Source: CAD feature listing. Evaluate the final solid. Frame: model axes, mm. A direction names the side the tool comes from. Round coordinates to 2 decimals unless told otherwise and drop trailing zeros. One line per item, written item: value.
Autodesk Inventor part; units mm, degrees
ref_plane "YZ Plane" through (0, 0, 0) normal (1, 0, 0) x (0, 1, 0)
ref_plane "XZ Plane" through (0, 0, 0) normal (0, 1, 0) x (-1, 0, 0)
ref_plane "XY Plane" through (0, 0, 0) normal (0, 0, 1) x (1, 0, 0)
sketch "_____4" plane through (0, 0, 0) normal (0, 0, 1) x (1, 0, 0)
  line L0 (-10, -3) -> (-10, -9)
  arc A0 (-10, -9) -> (-9, -10) centre (-9, -9) ccw
  line L1 (-9, -10) -> (-3, -10)
  line L2 (-3, -10) -> (-3, -8)
  line L3 (-3, -8) -> (-6, -8)
  line L4 (-6, -8) -> (-6, -7.0607)
  line L5 (-6, -7.0607) -> (-2.9393, -4)
  line L6 (-2.9393, -4) -> (-0.6536, -4)
  arc A1 (-0.6536, -4) -> (-0.4036, -3.933) centre (-0.6536, -3.5) ccw
  line L7 (-0.4036, -3.933) -> (0, -3.7)
  line L8 (0, -3.7) -> (0.4036, -3.933)
  arc A2 (0.4036, -3.933) -> (0.9036, -3.933) centre (0.6536, -3.5) ccw
  line L9 (0.9036, -3.933) -> (1.2189, -3.751)
  line L10 (1.2189, -3.751) -> (2.5, -4)
  line L11 (2.5, -4) -> (2.9393, -4)
  line L12 (2.9393, -4) -> (6, -7.0607)
  line L13 (6, -7.0607) -> (6, -8)
  line L14 (6, -8) -> (3, -8)
  line L15 (3, -8) -> (3, -10)
  line L16 (3, -10) -> (9, -10)
  arc A3 (9, -10) -> (10, -9) centre (9, -9) ccw
  line L17 (10, -9) -> (10, -3)
  line L18 (10, -3) -> (8, -3)
  line L19 (8, -3) -> (8, -6)
  line L20 (8, -6) -> (7.0607, -6)
  line L21 (7.0607, -6) -> (4, -2.9393)
  line L22 (4, -2.9393) -> (4, -0.6536)
  arc A4 (4, -0.6536) -> (3.933, -0.4036) centre (3.5, -0.6536) ccw
  line L23 (3.933, -0.4036) -> (3.7, 0)
  line L24 (3.7, 0) -> (3.933, 0.4036)
  arc A5 (3.933, 0.4036) -> (3.933, 0.9036) centre (3.5, 0.6536) ccw
  line L25 (3.933, 0.9036) -> (3.751, 1.2189)
  line L26 (3.751, 1.2189) -> (4, 2.5)
  line L27 (4, 2.5) -> (4, 2.9393)
  line L28 (4, 2.9393) -> (7.0607, 6)
  line L29 (7.0607, 6) -> (8, 6)
  line L30 (8, 6) -> (8, 3)
  line L31 (8, 3) -> (10, 3)
  line L32 (10, 3) -> (10, 9)
  arc A6 (10, 9) -> (9, 10) centre (9, 9) ccw
  line L33 (9, 10) -> (3, 10)
  line L34 (3, 10) -> (3, 8)
  line L35 (3, 8) -> (6, 8)
  line L36 (6, 8) -> (6, 7.0607)
  line L37 (6, 7.0607) -> (2.9393, 4)
  line L38 (2.9393, 4) -> (0.6536, 4)
  arc A7 (0.6536, 4) -> (0.4036, 3.933) centre (0.6536, 3.5) ccw
  line L39 (0.4036, 3.933) -> (0, 3.7)
  line L40 (0, 3.7) -> (-0.4036, 3.933)
  arc A8 (-0.4036, 3.933) -> (-0.9036, 3.933) centre (-0.6536, 3.5) ccw
  line L41 (-0.9036, 3.933) -> (-1.2189, 3.751)
  line L42 (-1.2189, 3.751) -> (-2.5, 4)
  line L43 (-2.5, 4) -> (-2.9393, 4)
  line L44 (-2.9393, 4) -> (-6, 7.0607)
  line L45 (-6, 7.0607) -> (-6, 8)
  line L46 (-6, 8) -> (-3, 8)
  line L47 (-3, 8) -> (-3, 10)
  line L48 (-3, 10) -> (-9, 10)
  arc A9 (-9, 10) -> (-10, 9) centre (-9, 9) ccw
  line L49 (-10, 9) -> (-10, 3)
  line L50 (-10, 3) -> (-8, 3)
  line L51 (-8, 3) -> (-8, 6)
  line L52 (-8, 6) -> (-7.0607, 6)
  line L53 (-7.0607, 6) -> (-4, 2.9393)
  line L54 (-4, 2.9393) -> (-4, 0.6536)
  arc A10 (-4, 0.6536) -> (-3.933, 0.4036) centre (-3.5, 0.6536) ccw
  line L55 (-3.933, 0.4036) -> (-3.7, 0)
  line L56 (-3.7, 0) -> (-3.933, -0.4036)
  arc A11 (-3.933, -0.4036) -> (-3.933, -0.9036) centre (-3.5, -0.6536) ccw
  line L57 (-3.933, -0.9036) -> (-3.751, -1.2189)
  line L58 (-3.751, -1.2189) -> (-4, -2.5)
  line L59 (-4, -2.5) -> (-4, -2.9393)
  line L60 (-4, -2.9393) -> (-7.0607, -6)
  line L61 (-7.0607, -6) -> (-8, -6)
  line L62 (-8, -6) -> (-8, -3)
  line L63 (-8, -3) -> (-10, -3)
extrude "Extrusion1" add sketch "_____4" against normal blind 140
sketch "Sketch2" plane through (0, 0, -140) normal (0, 0, -1) x (-1, 0, 0)
  point P0 (0, 0)
hole "Hole1" at (0, 0, -140) direction (0, 0, 1) diameter 4.2 depth 4000
properties part number "KNFS5-2020-3" material "アルミニウム 6061"
1. Ray query, line 1 (X direction, y = 0, z = -87); line 2 (Y direction, x = -5.25, z = -28); line 3 (X direction, y = -3.25, z = -24). Return the intervals inside material, ascending. Write a range as [from, to].
Report:
line 1: x = [-3.7, -2.1], [2.1, 3.7]
line 2: y = [-10, -8], [-6.31, -4.19], [4.19, 6.31], [8, 10]
line 3: x = [-10, -8], [-4.31, 4.31], [8, 10]
2. Pin query (flat end, axial travel): pin 1 (1.1 mm diameter, centred on y = 2, z = -42, fed in from -X); pin 2 (0.7 mm diameter, centred on x = 2, z = -87, fed in from +Y); pin 3 (1.1 mm diameter, centred on y = -1.5, z = -66, fed in from +X). Return the tip coordinate at first contact, or that it passes through.
Report:
pin 1: stops at x = -4
pin 2: stops at y = 4
pin 3: stops at x = 4
3. Reachability of faces 1 (the face through (6, -10, -69)), 2 (the face through (-8, -5, -69)), 3 (the face through (-6, 10, -69)), 4 (the face through (-4, 2, -69)), 5 (the face through (4, -2, -69)) from +Z, -Z, +X, -X, +Y, -Y: full face, straight path, thin tool, end or side. Return the list, or none.
Report:
face 1: +Z, -Z, +X, -X, -Y
face 2: +Z, -Z
face 3: +Z, -Z, +X, -X, +Y
face 4: +Z, -Z, -X
face 5: +Z, -Z, +X
4. Pull-direction query (Y, two-part tool) for faces 6 (the face through (4.49, 5.55, -69.02)), 7 (the face through (-0.1, 2.4, 0)), 8 (the face through (-2, -4, -69)); classes: released by +Y, released by -Y, zero draft, split by the parting line, or undercut.
Report:
face 6: undercut
face 7: zero draft
face 8: released by -Y
